from build123d import *

# Parameters (mm, degrees)
SKETCH1_W               = 305
SKETCH1_H               = 65
BOSS_EXTRUDE1_DEPTH     = 3.175
CUT_EXTRUDE2_START      = -3.175
SKETCH4_R               = 2.5
CUT_EXTRUDE2_DEPTH      = 6.35
CUT_EXTRUDE3_DEPTH      = 157.053908955
CUT_EXTRUDE3_DEPTH_BACK = 157.053908955
SKETCH5_R               = 2.5


with BuildPart() as part:
    # Sketch1 → Boss-Extrude1 (new, symmetric)
    with BuildSketch(Plane(origin=(0, 0, 0), x_dir=(1, 0, 0), z_dir=(0, 1, 0))):
        Rectangle(SKETCH1_W, SKETCH1_H)
    extrude(amount=BOSS_EXTRUDE1_DEPTH, both=True)

    # Sketch4 → Cut-Extrude2 (cut)
    with BuildSketch(Plane(origin=(-2.5, 0, 0), x_dir=(-1, 0, 0), z_dir=(0, -1, 0)).offset(CUT_EXTRUDE2_START)):
        with Locations(Location((133.48, -15.98, 0), (0, 0, 90))):
            Circle(SKETCH4_R)
        with Locations(Location((133.48, 15.98, 0), (0, 0, 270))):
            Circle(SKETCH4_R)
    cut_extrude2 = extrude(amount=CUT_EXTRUDE2_DEPTH, mode=Mode.SUBTRACT)

    # Mirror2: Cut-Extrude2 across plane
    add(cut_extrude2.mirror(Plane(origin=(0, 0, 0), x_dir=(0, 0, 1), z_dir=(1, 0, 0))), mode=Mode.SUBTRACT)

    # Sketch5 → Cut-Extrude3 (cut, two sides: drawn at the far end of the back side and taken through both)
    with BuildSketch(Plane(origin=(0, 3.175, 0), x_dir=(1, 0, 0), z_dir=(0, 1, 0)).offset(-CUT_EXTRUDE3_DEPTH_BACK)):
        with Locations(Location((122.5, 22.5, 0), (0, 0, 270))):
            Circle(SKETCH5_R)
        with Locations(Location((67.5, 22.5, 0), (0, 0, 270))):
            Circle(SKETCH5_R)
        with Locations(Location((142.5, 0, 0), (0, 0, 270))):
            Circle(SKETCH5_R)
    extrude(amount=CUT_EXTRUDE3_DEPTH + CUT_EXTRUDE3_DEPTH_BACK, mode=Mode.SUBTRACT)


solid = part.part
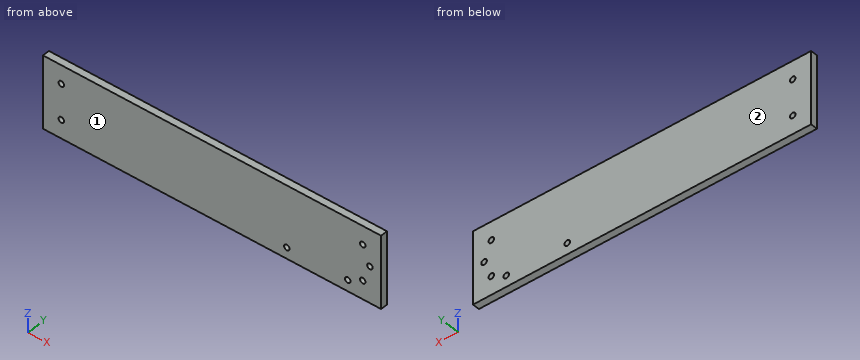
Can you work these out from the model? Positions are in its coordinate system, mm. Face numbers are marked on the shaded views. Coordinates: 2 decimals unless noted, no trailing zeros. Order: outer loops, then holes, each group sorted by start corner. A loop starts at its lowest first (then second) coordinate and runs counter-clockwise, first axis right, second up. Notation, with made-up numbers: M -34.5,62 L -7.5,62 A20 cw -7.5,68 Z; hole C 37,70 d7. An arc over 180 degrees is marked long. Write item = value, one per line.
(1) Suppose I cut it at D-D on z = 15.98. Please give me the cut outline in (x, y) (3 decimals).
Results are:
outline = M -152.5,-3.175 L -138.48,-3.175 L -138.48,3.175 L -152.5,3.175 Z; M -133.48,-3.175 L 133.48,-3.175 L 133.48,3.175 L -133.48,3.175 Z; M 138.48,-3.175 L 152.5,-3.175 L 152.5,3.175 L 138.48,3.175 Z
(2) Suppose I cut it at C-C on x = 122.5. Please give me the cut outline in (y, z) (3 decimals).
Results are:
outline = M -3.175,-32.5 L 3.175,-32.5 L 3.175,-25 L -3.175,-25 Z; M -3.175,-20 L 3.175,-20 L 3.175,32.5 L -3.175,32.5 Z
(3) I need wall thicknesses on line 1 along X through (y, z) = (2.75, -15.5); line 2 along X through (y, z) = (0.75, 15.98); line 3 along Z through (x, y) = (135.98, 1.5). Which ranges of each line are inside material? Lowest first, please. Write a range as [from, to].
Results are:
line_1 = [-152.5, -138.43], [-133.53, 133.53], [138.43, 152.5]
line_2 = [-152.5, -138.48], [-133.48, 133.48], [138.48, 152.5]
line_3 = [-32.5, -18.48], [-13.48, 13.48], [18.48, 32.5]
(4) If we mould it in two halves opening along Y, with no side actions, what happens to the marked faces 1 and 2? For each: pulls with the +Y half, pulls with the -Y half, needs draft (parallel to the pull), parting line crosses it, or undercut.
Results are:
face_1 = pulls with the -Y half
face_2 = pulls with the +Y half
(5) Suppose I cut it at A-A on z = 0. Please give me the cut outline in (x, y) (3 decimals).
Results are:
outline = M -152.5,-3.175 L 140,-3.175 L 140,3.175 L -152.5,3.175 Z; M 145,-3.175 L 152.5,-3.175 L 152.5,3.175 L 145,3.175 Z
(6) Suppose I cut it at B-B on x = -135.98. Please give me the cut outline in (y, z) (3 decimals).
Results are:
outline = M -3.175,-32.5 L 3.175,-32.5 L 3.175,-18.48 L -3.175,-18.48 Z; M -3.175,-13.48 L 3.175,-13.48 L 3.175,13.48 L -3.175,13.48 Z; M -3.175,18.48 L 3.175,18.48 L 3.175,32.5 L -3.175,32.5 Z
